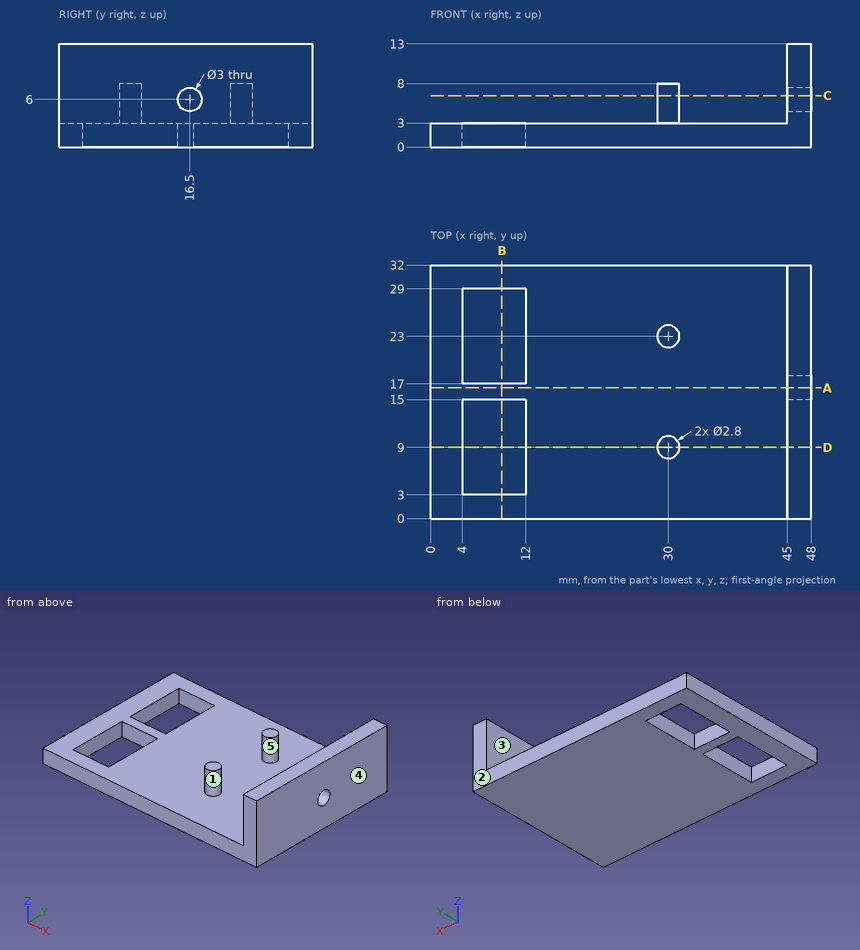
Job drawing, mm, ordinate dimensions from the low corner. One solid piece. A direction names the side the tool comes from. Give positions to 0.01 mm unless a question says otherwise; leave off trailing zeros. Order: outer loops, then holes, each group sorted by start corner. A loop starts at its lowest first (then second) coordinate and runs counter-clockwise, first axis right, second up. Notation, with made-up numbers: (17, 36) - (62, 36) arc R23 ccw to (62, 47) - close; hole circle Ø5 at (31, 61.5). An arc over 180 degrees is marked (long way). One line per question, with ' | ' between items.
1. Band-saw the part on D-D on y = 9. List the corners of the cut face in (x, z), then the cut area to 3 significant figures.
Filled in:
outline: (0, 0) - (4, 0) - (4, 3) - (0, 3) - close; (12, 0) - (48, 0) - (48, 13) - (45, 13) - (45, 3) - (31.4, 3) - (31.4, 8) - (28.6, 8) - (28.6, 3) - (12, 3) - close | area: 164 mm²
2. Band-saw the part on A-A on y = 16.5. List the corners of the cut face in (x, z).
Filled in:
outline: (0, 0) - (48, 0) - (48, 4.5) - (45, 4.5) - (45, 3) - (0, 3) - close; (45, 7.5) - (48, 7.5) - (48, 13) - (45, 13) - close
3. Band-saw the part on B-B on x = 9. List the corners of the cut face in (y, z), then the cut area to 3 significant figures.
Filled in:
outline: (0, 0) - (3, 0) - (3, 3) - (0, 3) - close; (15, 0) - (17, 0) - (17, 3) - (15, 3) - close; (29, 0) - (32, 0) - (32, 3) - (29, 3) - close | area: 24.0 mm²
4. Drop flat-ended pins along their axis: P1, Ø1.5, axis at x = 11, y = 14, coming from the +Z side; P2, Ø2, axis at x = 22, y = 13.5, coming from the +Z side; P3, Ø0.8, axis at x = 29.5, y = 9, coming from the +Z side. Give the stop position or say it passes through.
Filled in:
P1: through | P2: z = 3 | P3: z = 8
5. Band-saw the part on C-C on z = 6.5. List the corners of the cut face in (x, y).
Filled in:
outline: circle Ø2.8 at (30, 9); circle Ø2.8 at (30, 23); (45, 0) - (48, 0) - (48, 15.09) - (45, 15.09) - close; (45, 17.91) - (48, 17.91) - (48, 32) - (45, 32) - close
6. Which spindle directions (+Z, -Z, +X, -X, +Y, -Y) get a long thin tool onto all of the face, cutting with end or side? Do the marked faces 4 and 5. Say none if no direction does.
Filled in:
face 4: +Z, -Z, +X, +Y, -Y | face 5: +Z
7. Pull direction Y, two halves, no side cores. Call the marked faces 1, 2 and 3: +Y half, -Y half, draft (parallel to the pull), parting line (faces both ways), or undercut.
Filled in:
face 1: undercut | face 2: +Y half | face 3: draft
8. Drill centre lines: probe 1 along Y at (x, z) = (46.65, 6); probe 2 along Z at (x, y) = (45.8, 16.5); probe 3 along X at (y, z) = (11, 2.5). Where is each one in solid material? Low to high.
Filled in:
probe 1: 0 to 15, 18 to 32 | probe 2: 0 to 4.5, 7.5 to 13 | probe 3: 0 to 4, 12 to 48
